The listing builds one solid part. Answer for the finished solid, in the listing's coordinates (mm). A direction names the side the tool comes from. Round coordinates to 2 decimals unless told otherwise and drop trailing zeros. Write each loop counter-clockwise with the first axis right and the second up, starting at its lowest first coordinate (ties: lowest second). Pieces come first, ordered by that corner, then holes. Notation, with made-up numbers: (39.5, -7.75) - (69.5, -7.75) arc R20 ccw to (69.5, 9.25) - close; hole circle Ø1 at (-38.75, -32). An arc over 180 degrees is marked (long way). Return JSON: item names as keys, results as strings. Group by question number.
(1) Find the intervals of material crossed by line 1 along Y through (x, z) = (15.5, 29); line 2 along Z through (x, y) = (25, 0.25); line 3 along Z through (x, y) = (32.5, 1), in increasing order. Write a range as [from, to].
(2) Section B-B, the plane z = 5.5 is taken. Write down the section's boundary in (x, y), then the cut area to 3 significant figures.
(3) Determine the mould class of faces 1 (the flat face through (50, 0, 23)), 2 (the flat face through (12, -5, 39)), 3 (the flat face through (25, 10, 32)) for opening direction Y: +Y half, -Y half, draft (parallel to the pull), parting line (faces both ways), or undercut.
(4) Which of the six approach directions +Z, -Z, +X, -X, +Y, -Y give full straight-line access (tool end or side, diameter ignored) to faces 4 (the flat face through (5, 7, 47.16)), 5 (the flat face through (41, 0, 60.316)), 6 (the flat face through (12, 5, 39)), 7 (the flat face through (45, 0, 47.16)), 8 (the flat face through (20, 0, 25))?
(5) Each of these flat-tipped pins is pushed along its axis until it touches: pin 1 (13.5 mm diameter, centred on x = 21, z = 57, fed in from +Y); pin 2 (4 mm diameter, centred on x = 4.5, y = 8, fed in from +Z); pin 3 (5 mm diameter, centred on y = 6.5, z = 61, fed in from -X); pin 4 (1 mm diameter, centred on y = -5, z = 70, fed in from +X). Where does it stop, or does it pass through?
(6) Section C-C, the plane y = -7.5 is taken. Write down the section's boundary in (x, z), then the cut area to 3 significant figures.
(7) Section A-A, the plane x = 25 is taken. Write down the section's boundary in (y, z).
(8) Section D-D, the plane x = 6 is taken. Write down the section's boundary in (y, z) (3 decimals), then the cut area to 3 significant figures.
```python
from build123d import *

# Parameters (mm, degrees)
F0_R     = 12.5
F1_DEPTH = 10
F2_W     = 10
F2_H     = 90.439778
F3_DEPTH = 20
F5_DEPTH = 30.001


with BuildPart() as f1:
    # F0 (on Front) → F1 (new body, symmetric)
    with BuildSketch(Plane.XZ):
        with BuildLine():
            Line((0, 47.159518), (0, 0))
            Line((0, 0), (50, 0))
            Line((50, 0), (50, 47.159518))
            Line((50, 47.159518), (40.333689, 47.159518))
            ThreePointArc((40.333689, 47.159518), (25, 80), (9.666311, 47.159518))
            Line((9.666311, 47.159518), (0, 47.159518))
        make_face()
        with Locations((25, 60)):
            Circle(F0_R, mode=Mode.SUBTRACT)
    extrude(amount=F1_DEPTH, both=True)

    # F2 (on face) → F3 (cut, symmetric)
    with BuildSketch(Plane(origin=(0, 0, 0), x_dir=(0, -1, 0), z_dir=(-1, 0, 0))):
        with Locations((0, 45.219889)):
            Rectangle(F2_W, F2_H)
    extrude(amount=F3_DEPTH, both=True, mode=Mode.SUBTRACT)

    # F4 (on face) → F5 (cut, through all)
    with BuildSketch(Plane(origin=(20, 0, 0), x_dir=(0, -1, 0), z_dir=(-1, 0, 0))):
        Polygon((5, 84.635349), (-5, 81.45997), (-5, 71.508407), (-5, 60.315875), (5, 60.315875), (5, 71.456439), align=None)
    extrude(amount=-F5_DEPTH, mode=Mode.SUBTRACT)


solid = f1.part
```
Working result:
{
 "1": {"line 1": "y = [-10, -5], [5, 10]", "line 2": "z = [0, 47.5]", "line 3": "z = [0, 50]"},
 "2": {"outline": "(0, -10) - (50, -10) - (50, 10) - (0, 10) - (0, 5) - (20, 5) - (20, -5) - (0, -5) - close", "area": "800 mm^2"},
 "3": {"face 1": "draft", "face 2": "undercut", "face 3": "+Y half"},
 "4": {"face 4": "-X, +Y, -Y", "face 5": "+Z, +X, -X", "face 6": "+Z, -X", "face 7": "+X, +Y, -Y", "face 8": "+Z, -Z, -X"},
 "5": {"pin 1": "passes through", "pin 2": "stops at z = 67.6", "pin 3": "stops at x = 5", "pin 4": "stops at x = 42.6"},
 "6": {"outline": "(0, 0) - (50, 0) - (50, 47.16) - (40.33, 47.16) arc R20 ccw (long way) to (9.67, 47.16) - (0, 47.16) - close; hole circle Ø25 at (25, 60)", "area": "2,970 mm^2"},
 "7": {"outline": "(-10, 0) - (10, 0) - (10, 47.5) - (-10, 47.5) - close; (-10, 72.5) - (-5, 72.5) - (-5, 80) - (-10, 80) - close; (5, 72.5) - (10, 72.5) - (10, 80) - (5, 80) - close"},
 "8": {"outline": "(-10, 0) - (-5, 0) - (-5, 47.16) - (-10, 47.16) - close; (-10, 53.755) - (-5, 53.755) - (-5, 66.245) - (-10, 66.245) - close; (5, 0) - (10, 0) - (10, 47.16) - (5, 47.16) - close; (5, 53.755) - (10, 53.755) - (10, 66.245) - (5, 66.245) - close", "area": "596 mm^2"}
}
